Can you work these out from the model? Positions are in its coordinate system, mm. Face numbers are marked on the shaded views. Round coordinates to 2 decimals unless told otherwise and drop trailing zeros. Loops run counter-clockwise (first coordinate to the right, second up) from the corner with the lowest first, then second, coordinate; pieces in that order, holes last. Notation, with made-up numbers: (18.5, 43) -> (64.5, 43) arc R18 ccw to (64.5, 56) -> close; hole circle Ø8 at (72.25, 12.25). An arc over 180 degrees is marked (long way). Write item = value, one per line.
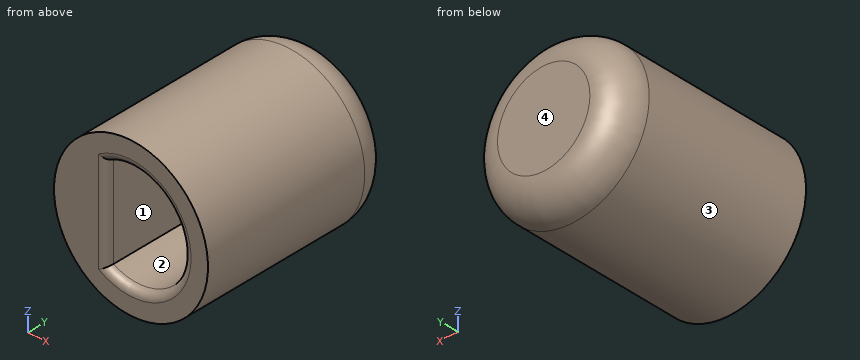
from build123d import *

# Parameters (mm, degrees)
SKETCH1_R           = 5
BOSS_EXTRUDE1_DEPTH = 13
CUT_EXTRUDE1_DEPTH  = 12.5
FILLET4_R           = 2
FILLET5_R           = 0.5
ROUND_BODY_R        = 2


with BuildPart() as part:
    # Sketch1 → Boss-Extrude1 (new body)
    with BuildSketch(Plane(origin=(0, 0, 0), x_dir=(1, 0, 0), z_dir=(0, 1, 0))):
        with Locations(Location((0, 0, 0), (0, 0, 90))):
            Circle(SKETCH1_R)
    extrude(amount=BOSS_EXTRUDE1_DEPTH)

    # Insert → Cut-Extrude1 (cut)
    with BuildSketch(Plane.XZ):
        with BuildLine():
            Line((-1.6, 3), (-1.6, -3))
            ThreePointArc((-1.6, -3), (3.4, 0), (-1.6, 3))
        make_face()
    extrude(amount=-CUT_EXTRUDE1_DEPTH, mode=Mode.SUBTRACT)

    # Fillet4
    # the kernel refuses this fillet: 2 mm, written as the material it adds along each edge
    with BuildSketch(Plane(origin=(0, 12.5, 0), x_dir=(-0.9999950652018581, 0, -0.003141587485880304), z_dir=(-0.003141587485880304, 0, 0.9999950652018581))) as fillet4_piece_1:
        with BuildLine():
            CenterArc((3.4 - FILLET4_R, FILLET4_R), FILLET4_R, 270, 90)
            Line((3.4 - FILLET4_R, 0), (3.4, 0))
            Line((3.4, 0), (3.4, FILLET4_R))
        make_face()
    revolve(axis=Axis((0, 12.5, 0), (0, -1, 0)), revolution_arc=359.64)
    with BuildSketch(Plane(origin=(-1.6, 12.5, 8), x_dir=(0, -1, 0), z_dir=(0, 0, -1))) as fillet4_piece_2_section:
        with BuildLine():
            CenterArc((FILLET4_R, -FILLET4_R), FILLET4_R, 90, 90)
            Line((0, -FILLET4_R), (0, 0))
            Line((0, 0), (FILLET4_R, 0))
        make_face()
    fillet4_piece_2 = extrude(amount=16, mode=Mode.PRIVATE)
    fillet4_piece_2 = fillet4_piece_2 & Plane(origin=(0, 12.061767945, 0), x_dir=(-0.4705882352941176, 0, -0.8823529411764707), z_dir=(0, -1, 0)) * Cylinder(3.4, 40, mode=Mode.PRIVATE)
    add(fillet4_piece_2)

    # Fillet5
    fillet5_edges = [part.edges().sort_by_distance(p)[0] for p in [
        (3.4, 0, 0),
        (-1.6, 0, 0),
    ]]
    fillet(fillet5_edges, radius=FILLET5_R)

    # Round Body
    round_body_edges = [part.edges().sort_by_distance(p)[0] for p in [
        (0, 13, 5),
    ]]
    fillet(round_body_edges, radius=ROUND_BODY_R)


solid = part.part
1. We'd pull the mould along X, two halves only. Please class the marked faces 1, 2, 3 and 4: released by +X, released by -X, zero draft, split by the parting line, or undercut.
Entries:
face_1 = undercut
face_2 = undercut
face_3 = split by the parting line
face_4 = zero draft
2. Suppose I cut it at A-A, the plane y = 1.75. List the corners of the cut face in (x, z) for me, and give its area (3 significant figures).
Entries:
outline = circle Ø10 at (0, 0); hole (-1.6, -3) arc R3.4 ccw (long way) to (-1.6, 3) -> close
area = 49.9 mm²
3. I need wall thicknesses on line 1 (Z direction, x = 0.75, y = 6.25); line 2 (X direction, y = 8.5, z = -2.5); line 3 (X direction, y = 7.5, z = 2.25). Which ranges of each line are inside material? Lowest first, please. Write a range as [from, to].
Entries:
line_1 = [-4.94, -3.32], [3.32, 4.94]
line_2 = [-4.33, -1.6], [2.3, 4.33]
line_3 = [-4.47, -1.6], [2.55, 4.47]
4. I'm going to push flat-ended pins straight in: pin 1 (2 mm diameter, centred on x = 4, y = 6.5, fed in from -Z); pin 2 (6 mm diameter, centred on x = -3.5, y = 4, fed in from +Z); pin 3 (2 mm diameter, centred on y = 7.5, z = 1.5, fed in from -X). Where does each tip first touch, or does it pass through?
Entries:
pin_1 = -4
pin_2 = 4.97
pin_3 = -4.97
